Autodesk Inventor part; units mm, degrees
ref_plane "YZ Plane" through (0, 0, 0) normal (1, 0, 0) x (0, 1, 0)
ref_plane "XZ Plane" through (0, 0, 0) normal (0, 1, 0) x (-1, 0, 0)
ref_plane "XY Plane" through (0, 0, 0) normal (0, 0, 1) x (1, 0, 0)
sketch "スケッチ1" plane through (0, 0, 0) normal (0, 0, 1) x (1, 0, 0)
  line L0 (0, 0) -> (6, 0)
  line L1 (6, 0) -> (6, 30)
  line L2 (6, 30) -> (0, 30)
  line L3 (0, 30) -> (0, 0)
  dimension "d0" = 6
  dimension "d1" = 30
extrude "押し出し1" add sketch "スケッチ1" along normal blind 2
sketch "スケッチ2" plane through (0, 0, 2) normal (0, 0, 1) x (1, 0, 0)
  line L0 (6, 30) -> (0, 30)
  line L1 (6, 0) -> (6, 30)
  line L2 (0, 0) -> (6, 0)
  point P0 (3, 25)
  point P1 (3, 5)
  dimension "d4" = 5
  dimension "d5" = 3
  dimension "d6" = 3
  dimension "d7" = 5
hole "穴1" at (3, 25, 2) at (3, 5, 2) direction (0, 0, -1) diameter 3.2 end through all
sketch "スケッチ4" plane through (0, 0, 2) normal (0, 0, 1) x (1, 0, 0)
  line L0 (6, 30) -> (0, 30)
  line L1 (6, 0) -> (6, 30)
  line L2 (0, 30) -> (6, 30)
  line L3 (6, 30) -> (6, 28)
  line L4 (6, 28) -> (0, 28)
  line L5 (0, 28) -> (0, 30)
  line L6 (0, 30) -> (0, 0)
  line L7 (0, 2) -> (6, 2)
  line L8 (6, 2) -> (6, 0)
  line L9 (6, 0) -> (0, 0)
  line L10 (0, 0) -> (0, 2)
  dimension "d18" = 2
  dimension "d19" = 2
extrude "押し出し2" cut sketch "スケッチ4" against normal blind 10 contours L1 L4 L5 L0 | L1 L9 L6 L7
sketch "スケッチ5" plane through (0, 0, 2) normal (0, 0, 1) x (1, 0, 0)
  line L0 (0, 28) -> (0, 2)
  line L1 (0, 27) -> (1, 28)
  line L2 (0, 28) -> (6, 28)
  line L3 (5, 28) -> (6, 27)
  line L4 (6, 2) -> (6, 28)
  point P0 (0, 0)
  dimension "d22" = 1
  dimension "d23" = 1
  dimension "d24" = 1
  dimension "d25" = 1
sketch "スケッチ6" plane through (0, 0, 2) normal (0, 0, 1) x (1, 0, 0)
  line L0 (0, 28) -> (0, 2)
  line L1 (0, 3) -> (1, 2)
  line L2 (6, 2) -> (0, 2)
  line L3 (6, 2) -> (6, 28)
  line L4 (6, 3) -> (5, 2)
  point P0 (0, 0)
  dimension "d26" = 1
  dimension "d27" = 1
  dimension "d28" = 1
  dimension "d29" = 1
extrude "押し出し3" cut sketch "スケッチ6" against normal blind 10
extrude "押し出し4" cut sketch "スケッチ5" against normal blind 10
properties part number "リンク26×6×2"
The model under review builds one solid part; all positions refer to its coordinate system, in mm. Give positions to 0.01 mm unless a question says otherwise; leave off trailing zeros. Loops run counter-clockwise (first coordinate to the right, second up) from the corner with the lowest first, then second, coordinate; pieces in that order, holes last. Notation, with made-up numbers: (-40, -9.5) -> (18, -9.5) arc R17 ccw to (18, 8.5) -> close; hole circle Ø3 at (66.25, 86.25). An arc over 180 degrees is marked (long way). Put each result on its own line as item: value. Start each with the question number.
1. We need section B-B on z = 0.6. State the section outline as (x, y) points, then the cut area to 3 significant figures.
2. We need section C-C on x = 3. State the section outline as (y, z) points, then the cut area to 3 significant figures.
3. Clearance check with a flat-ended pin moving along its axis: P1, Ø3, axis at x = 3, y = 25, coming from the +Z side. State where the tip first meets the part, or that it passes through.
4. We need section D-D on x = 5.55. State the section outline as (y, z) points.
5. We need section A-A on y = 5. State the section outline as (x, z) points.
6. Mouldability with a two-part tool opening along X and no side actions: class faces 1 (the face through (5.5, 2.5, 1)), 2 (the face through (3, 2, 1)), 3 (the face through (1.92, 26.18, 0.99)), 4 (the face through (0, 15, 1)) as released by +X, released by -X, zero draft, split by the parting line, or undercut.
7. Wall thickness on probe 1 along Y at (x, z) = (3, 1.2); probe 2 along Y at (x, z) = (3.65, 1.7); probe 3 along X at (y, z) = (25, 1.1): over which ranges is each line inside the solid? List them lowest first.
Determined:
1. outline: (0, 3) -> (1, 2) -> (5, 2) -> (6, 3) -> (6, 27) -> (5, 28) -> (1, 28) -> (0, 27) -> close; hole circle Ø3.2 at (3, 5); hole circle Ø3.2 at (3, 25)
1. area: 138 mm^2
2. outline: (2, 0) -> (3.4, 0) -> (3.4, 2) -> (2, 2) -> close; (6.6, 0) -> (23.4, 0) -> (23.4, 2) -> (6.6, 2) -> close; (26.6, 0) -> (28, 0) -> (28, 2) -> (26.6, 2) -> close
2. area: 39.2 mm^2
3. P1: through
4. outline: (2.55, 0) -> (27.45, 0) -> (27.45, 2) -> (2.55, 2) -> close
5. outline: (0, 0) -> (1.4, 0) -> (1.4, 2) -> (0, 2) -> close; (4.6, 0) -> (6, 0) -> (6, 2) -> (4.6, 2) -> close
6. face 1: released by +X
6. face 2: zero draft
6. face 3: undercut
6. face 4: released by -X
7. probe 1: 2 to 3.4, 6.6 to 23.4, 26.6 to 28
7. probe 2: 2 to 3.54, 6.46 to 23.54, 26.46 to 28
7. probe 3: 0 to 1.4, 4.6 to 6
